```python
from build123d import *

# Parameters (mm, degrees)
CROQUIS1_W              = 42.6
CROQUIS1_H              = 17.6
SALIENTE_EXTRUIR1_DEPTH = 24
CROQUIS2_R              = 1.2
CORTAR_EXTRUIR1_DEPTH   = 24
CROQUIS4_R              = 1.2
CORTAR_EXTRUIR2_DEPTH   = 10


with BuildPart() as part:
    # Croquis1 → Saliente-Extruir1 (new body)
    with BuildSketch(Plane.XY):
        Rectangle(CROQUIS1_W, CROQUIS1_H)
    extrude(amount=SALIENTE_EXTRUIR1_DEPTH)

    # Croquis2 → Cortar-Extruir1 (cut)
    with BuildSketch(Plane(origin=(0, 8.8, 0), x_dir=(1, 0, 0), z_dir=(0, 1, 0))):
        with Locations((-12, -6)):
            Circle(CROQUIS2_R)
        with Locations((12, -6)):
            Circle(CROQUIS2_R)
    extrude(amount=-CORTAR_EXTRUIR1_DEPTH, mode=Mode.SUBTRACT)

    # Croquis4 → Cortar-Extruir2 (cut)
    with BuildSketch(Plane.XY.offset(24)):
        with Locations((-14, 0)):
            Circle(CROQUIS4_R)
        with Locations((-5, 5)):
            Circle(CROQUIS4_R)
        with Locations((5, 5)):
            Circle(CROQUIS4_R)
        with Locations((14, 0)):
            Circle(CROQUIS4_R)
        with Locations((5, -5)):
            Circle(CROQUIS4_R)
        with Locations((-5, -5)):
            Circle(CROQUIS4_R)
    extrude(amount=-CORTAR_EXTRUIR2_DEPTH, mode=Mode.SUBTRACT)


solid = part.part
```
CAD build for the part. Positions are in the model's coordinates, mm. A direction names the side the tool comes from. Give positions to 0.01 mm unless a question says otherwise; leave off trailing zeros. Loops run counter-clockwise (first coordinate to the right, second up) from the corner with the lowest first, then second, coordinate; pieces in that order, holes last. Notation, with made-up numbers: (-20, 32.25) -> (28, 32.25) arc R16 cw to (28, 61.25) -> close; hole circle Ø7 at (-35.5, 61). An arc over 180 degrees is marked (long way). Use a Markdown table: item, result.
1. Slice it at B-B (y = 0). List the corners of the cut face in (x, z).
Check result:
| item | result |
|---|---|
| outline | (-21.3, 0) -> (21.3, 0) -> (21.3, 24) -> (15.2, 24) -> (15.2, 14) -> (12.8, 14) -> (12.8, 24) -> (-12.8, 24) -> (-12.8, 14) -> (-15.2, 14) -> (-15.2, 24) -> (-21.3, 24) -> close; hole circle Ø2.4 at (-12, 6); hole circle Ø2.4 at (12, 6) |
2. Mould opens along X. For faces 1 (the flat face through (21.3, 0, 12)), 2 (the cylindrical face through (13.145, 0.123, 5.64)), 3 (the flat face through (0, 8.8, 12)) say: pulls with the +X half, pulls with the -X half, needs draft (parallel to the pull), parting line crosses it, or undercut.
Check result:
| item | result |
|---|---|
| face 1 | pulls with the +X half |
| face 2 | undercut |
| face 3 | needs draft |
3. Slice it at C-C (z = 5.25). List the corners of the cut face in (x, y).
Check result:
| item | result |
|---|---|
| outline | (-21.3, -8.8) -> (-12.94, -8.8) -> (-12.94, 8.8) -> (-21.3, 8.8) -> close; (-11.06, -8.8) -> (11.06, -8.8) -> (11.06, 8.8) -> (-11.06, 8.8) -> close; (12.94, -8.8) -> (21.3, -8.8) -> (21.3, 8.8) -> (12.94, 8.8) -> close |
4. Slice it at A-A (x = -12). List the corners of the cut face in (y, z).
Check result:
| item | result |
|---|---|
| outline | (-8.8, 0) -> (8.8, 0) -> (8.8, 4.8) -> (-8.8, 4.8) -> close; (-8.8, 7.2) -> (8.8, 7.2) -> (8.8, 24) -> (-8.8, 24) -> close |
5. Which spindle directions (+Z, -Z, +X, -X, +Y, -Y) get a long thin tool onto all of the face, cutting with end or side? Do faces 4 (the cylindrical face through (-6.2, 5.05, 19.07)), 5 (the flat face through (0, 0, 24)). Say none if no direction does.
Check result:
| item | result |
|---|---|
| face 4 | +Z |
| face 5 | +Z, +X, -X, +Y, -Y |
6. Flat gauge pin, fed straight in: pin 1 (0.7 mm diameter, centred on x = -14.5, y = 0, fed in from +Z). Where does the tip first touch, or does it go through?
Check result:
| item | result |
|---|---|
| pin 1 | stops at z = 14 |
7. Wall check: L1, parallel to Y at x = -5, z = 19.75; L2, parallel to X at y = -2, z = 6; L3, parallel to Y at x = -4, z = 19. Give the ranges that are in metal, low to high. Write a range as [from, to].
Check result:
| item | result |
|---|---|
| L1 | y = [-8.8, -6.2], [-3.8, 3.8], [6.2, 8.8] |
| L2 | x = [-21.3, -13.2], [-10.8, 10.8], [13.2, 21.3] |
| L3 | y = [-8.8, -5.66], [-4.34, 4.34], [5.66, 8.8] |
8. Slice it at D-D (x = 14). List the corners of the cut face in (y, z), plus the area to 3 significant figures.
Check result:
| item | result |
|---|---|
| outline | (-8.8, 0) -> (8.8, 0) -> (8.8, 24) -> (1.2, 24) -> (1.2, 14) -> (-1.2, 14) -> (-1.2, 24) -> (-8.8, 24) -> close |
| area | 398 mm^2 |
